```python
from build123d import *

# Parameters (mm, degrees)
F0_W      = 1200
F0_H      = 600
F1_DEPTH  = 250
F2_W      = 600
F2_H      = 600
F3_DEPTH  = 300
F4_R      = 200
F5_DEPTH  = 550.001
F6_W      = 300
F6_H      = 150
F7_DEPTH  = 300
F8_W      = 300
F8_H      = 150
F9_DEPTH  = 300
F11_DEPTH = 600.001
F13_DEPTH = 150.0010001
F15_DEPTH = 150.0010001
F16_R     = 50
F17_SIZE2 = 5
F17_SIZE  = 5


with BuildPart() as f1:
    # F0 (on Top) → F1 (new body)
    with BuildSketch(Plane.XY):
        Rectangle(F0_W, F0_H)
    extrude(amount=F1_DEPTH)

    # F2 (on face) → F3 (join)
    with BuildSketch(Plane.XY.offset(250)):
        Rectangle(F2_W, F2_H)
    extrude(amount=F3_DEPTH)

    # F4 (on face) → F5 (cut, through all)
    with BuildSketch(Plane.XY.offset(550)):
        Circle(F4_R)
    extrude(amount=-F5_DEPTH, mode=Mode.SUBTRACT)

    # F6 (on face) → F7 (join)
    with BuildSketch(Plane.XY.offset(250)):
        with Locations((450, 225)):
            Rectangle(F6_W, F6_H)
    extrude(amount=F7_DEPTH)

    # F8 (on face) → F9 (join)
    with BuildSketch(Plane.XY.offset(250)):
        with Locations((-450, 225)):
            Rectangle(F8_W, F8_H)
    extrude(amount=F9_DEPTH)

    # F10 (on face) → F11 (cut, through all)
    with BuildSketch(Plane.XZ.offset(300)):
        with BuildLine():
            ThreePointArc((50, 263.3974596216), (86.6025403784, 300), (100, 350))
            ThreePointArc((100, 350), (-50, 436.6025403784), (-50, 263.3974596216))
            ThreePointArc((-50, 263.3974596216), (0, 250), (50, 263.3974596216))
        make_face()
        with BuildLine():
            ThreePointArc((50, 263.3974596216), (0, 250), (-50, 263.3974596216))
            Line((-50, 263.3974596216), (-50, 0))
            Line((-50, 0), (50, 0))
            Line((50, 0), (50, 263.3974596216))
        make_face()
    extrude(amount=-F11_DEPTH, mode=Mode.SUBTRACT)

    # F12 (on face) → F13 (cut, through all)
    with BuildSketch(Plane.XZ.offset(-150)):
        Polygon((600, 550), (300, 550), (600, 250), align=None)
    extrude(amount=-F13_DEPTH, mode=Mode.SUBTRACT)

    # F14 (on face) → F15 (cut, through all)
    with BuildSketch(Plane.XZ.offset(-150)):
        Polygon((-600, 250), (-300, 550), (-600, 550), align=None)
    extrude(amount=-F15_DEPTH, mode=Mode.SUBTRACT)

    # F16
    f16_edges = [f1.edges().sort_by_distance(p)[0] for p in [
        (300, -75, 250),
    ]]
    fillet(f16_edges, radius=F16_R)

    # F17
    f17_edges = [f1.edges().sort_by_distance(p)[0] for p in [
        (0, -300, 550),
    ]]
    chamfer(f17_edges, length=F17_SIZE, length2=F17_SIZE2)


solid = f1.part
```
CAD build for the part. Positions are in the model's coordinates, mm. A direction names the side the tool comes from. Give positions to 0.01 mm unless a question says otherwise; leave off trailing zeros. Write each loop counter-clockwise with the first axis right and the second up, starting at its lowest first coordinate (ties: lowest second). Pieces come first, ordered by that corner, then holes. Notation, with made-up numbers: M -7.75,19 L 8.25,19 A17 cw 8.25,52 Z; hole C 56.25,-4.5 d9. An arc over 180 degrees is marked long. Return JSON: item names as keys, results as strings. Group by question number.
(1) Drill centre lines: L1, parallel to X at y = -212.5, z = 350; L2, parallel to Z at x = 0, y = 233; L3, parallel to Y at x = -56, z = 464.5. Where is each one in solid material? Low to high. Write a range as [from, to].
(2) Flat gauge pin, fed straight in: pin 1 Ø2 at (x, y) = (-255, 114.5) entering from -Z. Where does the tip first touch, or does it go through?
(3) Band-saw the part on C-C (x = 0). Give the cut face in (y, z).
(4) Band-saw the part on A-A (y = 0). Give the cut face in (x, z), and give its area (3 significant figures).
(5) Mould opens along X. For faces 1 (the face through (-452, -72, 250)), 2 (the face through (-300, -78, 398)), 3 (the face through (315.036, -71.85, 264.258)), 4 (the face through (190.764, 60.075, 278.85)) say: pulls with the +X half, pulls with the -X half, needs draft (parallel to the pull), parting line crosses it, or undercut.
(6) 3-axis set-ups, long thin cutter, end or side, ignore diameter. For faces 5 (the face through (-50, 246, 134)), 6 (the face through (-385, 150, 331)), 7 (the face through (415, 150, 365)): which of +Z, -Z, +X, -X, +Y, -Y reach the whole face in a straight line?
(7) Band-saw the part on D-D (y = -253). Give the cut face in (x, z), and give its area (3 significant figures).
(8) Band-saw the part on B-B (z = 193.5). Give the cut face in (x, y).
Entries:
{
 "1": {"L1": "x = [-300, -100], [100, 300]", "L2": "z = [450, 550]", "L3": "y = [-300, -192], [192, 300]"},
 "2": {"pin 1": "stops at z = 0"},
 "3": {"outline": "M -300,450 L -200,450 L -200,550 L -295,550 L -300,545 Z; M 200,450 L 300,450 L 300,550 L 200,550 Z"},
 "4": {"outline": "M -600,0 L -200,0 L -200,550 L -300,550 L -300,250 L -600,250 Z; M 200,0 L 600,0 L 600,250 L 350,250 A50 cw 300,300 L 300,550 L 200,550 Z", "area": "261,000 mm^2"},
 "5": {"face 1": "needs draft", "face 2": "pulls with the -X half", "face 3": "pulls with the +X half", "face 4": "undercut"},
 "6": {"face 5": "-Z, +Y, -Y", "face 6": "+Z, -X, -Y", "face 7": "+Z, +X, -Y"},
 "7": {"outline": "M -600,0 L -50,0 L -50,263.4 A100 cw long 50,263.4 L 50,0 L 600,0 L 600,250 L 350,250 A50 cw 300,300 L 300,550 L -300,550 L -300,250 L -600,250 Z", "area": "424,000 mm^2"},
 "8": {"outline": "M -600,-300 L -50,-300 L -50,-193.65 A200 cw -50,193.65 L -50,300 L -600,300 Z; M 50,-300 L 600,-300 L 600,300 L 50,300 L 50,193.65 A200 cw 50,-193.65 Z"}
}
